```python
from build123d import *

# Parameters (mm, degrees)
SKETCH1_R           = 2.15
BOSS_EXTRUDE1_DEPTH = 4
CHAMFER2_SIZE       = 2.3
CHAMFER3_SIZE       = 1


with BuildPart() as part:
    # Sketch1 → Boss-Extrude1 (new body)
    with BuildSketch(Plane.XY):
        Polygon((10, 10), (30, 10), (30, -10), (-30, -10), (-30, 10), (-10, 10), (-10, 50), (10, 50), align=None)
        with Locations((0, 20)):
            Circle(SKETCH1_R, mode=Mode.SUBTRACT)
        with Locations((20, 0)):
            Circle(SKETCH1_R, mode=Mode.SUBTRACT)
        with Locations((-20, 0)):
            Circle(SKETCH1_R, mode=Mode.SUBTRACT)
        with Locations((0, 40)):
            Circle(SKETCH1_R, mode=Mode.SUBTRACT)
        Circle(SKETCH1_R, mode=Mode.SUBTRACT)
    extrude(amount=BOSS_EXTRUDE1_DEPTH)

    # Chamfer2
    chamfer2_edges = [part.edges().sort_by_distance(p)[0] for p in [
        (17.85, 0, 4),
        (-2.15, 20, 4),
        (-22.15, 0, 4),
        (-2.15, 40, 4),
        (-2.15, 0, 4),
    ]]
    chamfer(chamfer2_edges, length=CHAMFER2_SIZE)

    # Chamfer3
    chamfer3_edges = [part.edges().sort_by_distance(p)[0] for p in [
        (10, 30, 4),
        (0, 50, 4),
        (-10, 30, 4),
        (-20, 10, 4),
        (-30, 0, 4),
        (0, -10, 4),
        (30, 0, 4),
        (20, 10, 4),
    ]]
    chamfer(chamfer3_edges, length=CHAMFER3_SIZE)


solid = part.part
```
For this review, take the finished solid that the model builds, in its own axes (mm). A direction names the side the tool comes from. Round coordinates to 2 decimals unless told otherwise and drop trailing zeros. Order: outer loops, then holes, each group sorted by start corner. A loop starts at its lowest first (then second) coordinate and runs counter-clockwise, first axis right, second up.
Q1. Mouldability with a two-part tool opening along X and no side actions: class faces 3 (the flat face through (0, 14, 4)), 4 (the cylindrical face through (-2.15, 0.09, 0.84)), 5 (the flat face through (30, 0, 1)) as pulls with the +X half, pulls with the -X half, needs draft (parallel to the pull), parting line crosses it, or undercut.
Findings below:
face 3: needs draft
face 4: undercut
face 5: pulls with the +X half
Q2. We need section C-C, the plane y = 0. Give the boundary of the cut face in (x, z).
Findings below:
outline: (-30, 0) - (-22.15, 0) - (-22.15, 1.7) - (-24.45, 4) - (-29, 4) - (-30, 3) - close; (-17.85, 0) - (-2.15, 0) - (-2.15, 1.7) - (-4.45, 4) - (-15.55, 4) - (-17.85, 1.7) - close; (2.15, 0) - (17.85, 0) - (17.85, 1.7) - (15.55, 4) - (4.45, 4) - (2.15, 1.7) - close; (22.15, 0) - (30, 0) - (30, 3) - (29, 4) - (24.45, 4) - (22.15, 1.7) - close
Q3. Insertion check: P1, Ø2, axis at y = 13.5, z = 3, coming from the +X side; P2, Ø5, axis at x = 0, y = 0, coming from the +Z side. Each pin has a flat end and moves straight along its axis. Give the tip position at first contact, or say it passes through.
Findings below:
P1: stops at x = 10
P2: stops at z = 2.05
Q4. Machinability: for faces 1 (the conical face through (1.23, 1.93, 1.84)), 2 (the flat face through (20, 10, 1)), which of the approach directions +Z, -Z, +X, -X, +Y, -Y give a long, thin tool a straight path to every point of the face, cutting with its end or side? Answer none if there is none.
Findings below:
face 1: +Z
face 2: +Z, -Z, +X, +Y
Q5. We need section D-D, the plane x = 0. Give the boundary of the cut face in (y, z), plus the area to 3 significant figures.
Findings below:
outline: (-10, 0) - (-2.15, 0) - (-2.15, 1.7) - (-4.45, 4) - (-9, 4) - (-10, 3) - close; (2.15, 0) - (17.85, 0) - (17.85, 1.7) - (15.55, 4) - (4.45, 4) - (2.15, 1.7) - close; (22.15, 0) - (37.85, 0) - (37.85, 1.7) - (35.55, 4) - (24.45, 4) - (22.15, 1.7) - close; (42.15, 0) - (50, 0) - (50, 3) - (49, 4) - (44.45, 4) - (42.15, 1.7) - close
area: 172 mm2
Q6. We need section A-A, the plane y = 20. Give the boundary of the cut face in (x, z), plus the area to 3 significant figures.
Findings below:
outline: (-10, 0) - (-2.15, 0) - (-2.15, 1.7) - (-4.45, 4) - (-9, 4) - (-10, 3) - close; (2.15, 0) - (10, 0) - (10, 3) - (9, 4) - (4.45, 4) - (2.15, 1.7) - close
area: 56.5 mm2
Q7. Wall thickness on line 1 (Y direction, x = 0, z = 0.7); line 2 (Y direction, x = -20, z = 0.65); line 3 (X direction, y = -2, z = 1.95): over which ranges is each line inside the solid? List them lowest first.
Findings below:
line 1: y = -10 to -2.15, 2.15 to 17.85, 22.15 to 37.85, 42.15 to 50
line 2: y = -10 to -2.15, 2.15 to 10
line 3: x = -30 to -21.33, -18.67 to -1.33, 1.33 to 18.67, 21.33 to 30
